```python
from build123d import *

# Parameters (mm, degrees)
MODEL_W             = 6
MODEL_H             = 6
BOSS_EXTRUDE1_DEPTH = 6


with BuildPart() as part:
    # Model → Boss-Extrude1 (new body)
    with BuildSketch(Plane.XY):
        with BuildLine():
            Line((3736.95412545, 1243.781770146), (3749.525554021, 1243.781770146))
            Line((3749.525554021, 1243.781770146), (3749.525554021, 1246.781770146))
            Line((3749.525554021, 1246.781770146), (3757.525554021, 1246.781770146))
            Line((3757.525554021, 1246.781770146), (3757.525554021, 1249.781770146))
            Line((3757.525554021, 1249.781770146), (3765.525554021, 1249.781770146))
            Line((3765.525554021, 1249.781770146), (3765.525554021, 1246.781770146))
            Line((3765.525554021, 1246.781770146), (3773.525554021, 1246.781770146))
            Line((3773.525554021, 1246.781770146), (3773.525554021, 1243.781770146))
            Line((3773.525554021, 1243.781770146), (3786.096982592, 1243.781770146))
            ThreePointArc((3786.096982592, 1243.781770146), (3761.525554021, 1268.353198718), (3736.95412545, 1243.781770146))
        make_face()
        with Locations((3774.525554021, 1256.781770147)):
            Rectangle(MODEL_W, MODEL_H, mode=Mode.SUBTRACT)
        with Locations((3748.525554021, 1256.781770147)):
            Rectangle(MODEL_W, MODEL_H, mode=Mode.SUBTRACT)
        with Locations((3761.525554021, 1256.781770147)):
            Rectangle(MODEL_W, MODEL_H, mode=Mode.SUBTRACT)
    extrude(amount=BOSS_EXTRUDE1_DEPTH)


solid = part.part
```
Read the model definition and answer for the solid it produces. Units are mm, in the model's axes. A direction names the side the tool comes from. Coordinates: 2 decimals unless noted, no trailing zeros. Order: outer loops, then holes, each group sorted by start corner. A loop starts at its lowest first (then second) coordinate and runs counter-clockwise, first axis right, second up. Notation, with made-up numbers: (28, 30.25) - (40, 30.25) arc R22 cw to (40, 54.25) - close; hole circle Ø10 at (8, -24). An arc over 180 degrees is marked (long way). Answer as a JSON object with one key per item and string values. Group by question number.
Item 1: Section B-B (y = 1249.25) is taken. Give the vertices of the cut face in (x, z), plus the area to 3 significant figures.
Item 2: Consider probe 1 along X at (y, z) = (1254.75, 3.9); probe 2 along Y at (x, z) = (3762, 3.9); probe 3 along X at (y, z) = (1258.5, 1.15). Determine where each line is inside the solid, lowest interval first. Write a range as from..to.
Item 3: Section C-C (x = 3762) is taken. Give the vertices of the cut face in (y, z), plus the area to 3 significant figures.
Item 4: Section D-D (y = 1258.25) is taken. Give the vertices of the cut face in (x, z), plus the area to 3 significant figures.
Item 5: Section A-A (z = 4.1) is taken. Give the vertices of the cut face in (x, y), plus the area to 3 significant figures.
Item 6: Flat-ended cylindrical pins translate along their axes: P1, Ø3, axis at x = 3765, z = 1.5, coming from the +Y side; P2, Ø3, axis at x = 3762.5, z = 2, coming from the +Y side; P3, Ø3, axis at x = 3748, z = 2, coming from the +Y side. Find the tip coordinate at first contact, or state that the pin passes through.
Item 7: A tool of negligible diameter and unlimited length cuts with its end or side. For faces 1 (the face through (3758.526, 1257, 3)), 2 (the face through (3761, 1249.782, 3)), 3 (the face through (3761.2, 1253.5, 0)), from which of +Z, -Z, +X, -X, +Y, -Y can it reach the whole face along a straight path? Write none if from no direction.
Item 8: The mould has two halves that part along Y. Classify faces 4 (the face through (3769, 1246.782, 3)), 5 (the face through (3777.526, 1257, 3)), 6 (the face through (3757.526, 1248, 3)): +Y half, -Y half, draft (parallel to the pull), parting line (faces both ways), or undercut.
Results are:
{
 "1": {"outline": "(3737.57, 0) - (3757.53, 0) - (3757.53, 6) - (3737.57, 6) - close; (3765.53, 0) - (3785.48, 0) - (3785.48, 6) - (3765.53, 6) - close", "area": "239 mm^2"},
 "2": {"probe 1": "x = 3739.54..3745.53, 3751.53..3758.53, 3764.53..3771.53, 3777.53..3783.51", "probe 2": "y = 1249.78..1253.78, 1259.78..1268.35", "probe 3": "x = 3741.85..3745.53, 3751.53..3758.53, 3764.53..3771.53, 3777.53..3781.2"},
 "3": {"outline": "(1249.78, 0) - (1253.78, 0) - (1253.78, 6) - (1249.78, 6) - close; (1259.78, 0) - (1268.35, 0) - (1268.35, 6) - (1259.78, 6) - close", "area": "75.4 mm^2"},
 "4": {"outline": "(3741.67, 0) - (3745.53, 0) - (3745.53, 6) - (3741.67, 6) - close; (3751.53, 0) - (3758.53, 0) - (3758.53, 6) - (3751.53, 6) - close; (3764.53, 0) - (3771.53, 0) - (3771.53, 6) - (3764.53, 6) - close; (3777.53, 0) - (3781.39, 0) - (3781.39, 6) - (3777.53, 6) - close", "area": "130 mm^2"},
 "5": {"outline": "(3736.95, 1243.78) - (3749.53, 1243.78) - (3749.53, 1246.78) - (3757.53, 1246.78) - (3757.53, 1249.78) - (3765.53, 1249.78) - (3765.53, 1246.78) - (3773.53, 1246.78) - (3773.53, 1243.78) - (3786.1, 1243.78) arc R24.57 ccw to start; hole (3745.53, 1253.78) - (3751.53, 1253.78) - (3751.53, 1259.78) - (3745.53, 1259.78) - close; hole (3758.53, 1253.78) - (3764.53, 1253.78) - (3764.53, 1259.78) - (3758.53, 1259.78) - close; hole (3771.53, 1253.78) - (3777.53, 1253.78) - (3777.53, 1259.78) - (3771.53, 1259.78) - close", "area": "744 mm^2"},
 "6": {"P1": "stops at y = 1268.27", "P2": "stops at y = 1268.35", "P3": "stops at y = 1265.21"},
 "7": {"face 1": "+Z, -Z", "face 2": "+Z, -Z, -Y", "face 3": "-Z, +X, -X, +Y, -Y"},
 "8": {"face 4": "-Y half", "face 5": "undercut", "face 6": "draft"}
}
